from build123d import *

# Parameters (mm, degrees)
F0_W     = 220
F0_H     = 220
F0_R     = 1.5
F1_DEPTH = 5
F2_SIZE  = 2
F3_DEPTH = 15


with BuildPart() as f1:
    # F0 (on Top) → F1 (new body)
    with BuildSketch(Plane.XY):
        Rectangle(F0_W, F0_H)
        with Locations((-104.5, -104.5)):
            Circle(F0_R, mode=Mode.SUBTRACT)
        with Locations((104.5, -104.5)):
            Circle(F0_R, mode=Mode.SUBTRACT)
        with Locations((-104.5, 104.5)):
            Circle(F0_R, mode=Mode.SUBTRACT)
        with Locations((104.5, 104.5)):
            Circle(F0_R, mode=Mode.SUBTRACT)
    extrude(amount=-F1_DEPTH)

    # F2
    f2_edges = [f1.edges().sort_by_distance(p)[0] for p in [
        (-106, 104.5, 0),
        (103, 104.5, 0),
        (103, -104.5, 0),
        (-106, -104.5, 0),
    ]]
    chamfer(f2_edges, length=F2_SIZE)

    # F0 (on Top) → F3 (join)
    with BuildSketch(Plane.XY):
        with Locations((-104.5, 104.5)):
            Circle(F0_R)
        with Locations((-104.5, -104.5)):
            Circle(F0_R)
        with Locations((104.5, -104.5)):
            Circle(F0_R)
        with Locations((104.5, 104.5)):
            Circle(F0_R)
    extrude(amount=-F3_DEPTH)


solid = f1.part
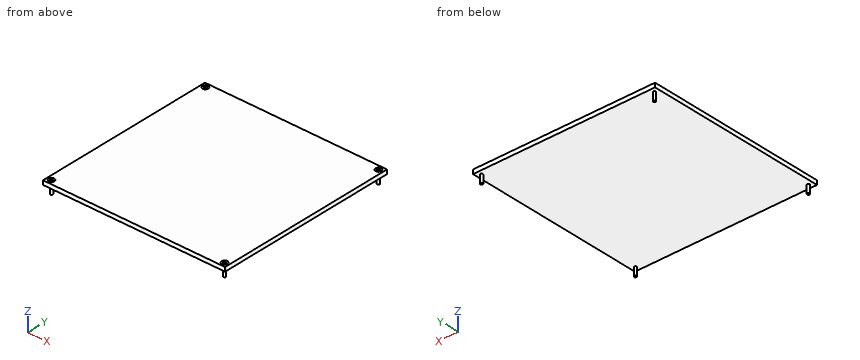
Could you check a few things on this model? Use its own coordinates, in mm. Coordinates: 2 decimals unless noted, no trailing zeros. Write each loop counter-clockwise with the first axis right and the second up, starting at its lowest first coordinate (ties: lowest second). Pieces come first, ordered by that corner, then holes. Notation, with made-up numbers: (-1.5, -25.75) - (21.5, -25.75) arc R33 ccw to (21.5, 5.25) - close; hole circle Ø10 at (16, 16.5). An arc over 180 degrees is marked (long way). Write item = value, one per line.
1) Suppose I cut it at A-A on z = -8.5. Please give me the cut outline in (x, y).
Result set:
outline = circle Ø3 at (-104.5, -104.5); circle Ø3 at (-104.5, 104.5); circle Ø3 at (104.5, -104.5); circle Ø3 at (104.5, 104.5)
2) Suppose I cut it at B-B on y = 41. Please give me the cut outline in (x, z), plus the area to 3 significant figures.
Result set:
outline = (-110, -5) - (110, -5) - (110, 0) - (-110, 0) - close
area = 1,100 mm2
3) Please list where this line runs through material, in increasing order: line 1 (Z direction, x = 94, y = 16). Write a range as [from, to].
Result set:
line_1 = [-5, 0]
4) Will these pins go through, and if not, where does the flat tip stop? pin 1 Ø1.5 at (x, y) = (46, -73.5) entering from -Z; pin 2 Ø8 at (x, y) = (-18, -2.5) entering from +Z.
Result set:
pin_1 = -5
pin_2 = 0
